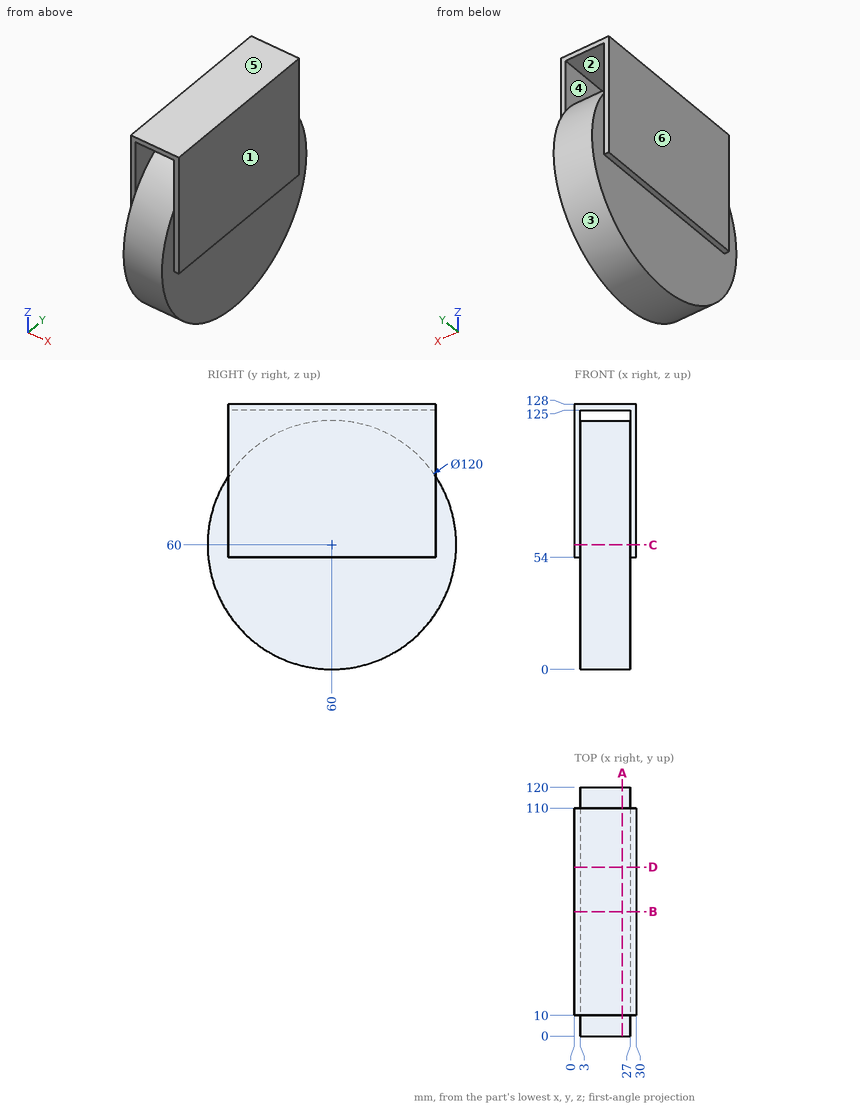
Design review of the part shown in the three views and the two pictorial views. Dimensions are in mm from the part's minimum x, y and z. A direction names the side the tool comes from. Give positions to 0.01 mm unless a question says otherwise; leave off trailing zeros. Write each loop counter-clockwise with the first axis right and the second up, starting at its lowest first coordinate (ties: lowest second). Pieces come first, ordered by that corner, then holes. Notation, with made-up numbers: (72.5, 22) - (81.5, 22) arc R19 ccw to (81.5, 30) - close; hole circle Ø10 at (74.25, 24.25). An arc over 180 degrees is marked (long way). Return JSON: item names as keys, results as strings. Group by question number.
(1) Insertion check: pin 1 (12 mm diameter, centred on x = 23.5, z = 107, fed in from -Y); pin 2 (8 mm diameter, centred on x = 24, y = 72.5, fed in from -Z); pin 3 (3.5 mm diameter, centred on x = 2, y = 54.5, fed in from -Z). Each pin has a flat end and moves straight along its axis. Give the tip position at first contact, or say it passes through.
(2) Mouldability with a two-part tool opening along X and no side actions: class the marked faces 4, 5 and 6 as +X half, -X half, draft (parallel to the pull), parting line (faces both ways), or undercut.
(3) We need section C-C, the plane z = 60. Give the boundary of the cut face in (x, y).
(4) We need section A-A, the plane x = 23.25. Give the boundary of the cut face in (y, z).
(5) Machinability: for the marked faces 1, 2 and 3, which of the approach directions +Z, -Z, +X, -X, +Y, -Y give a long, thin tool a straight path to every point of the face, cutting with its end or side? Answer none if there is none.
(6) We need section B-B, the plane y = 60. Give the boundary of the cut face in (x, z).
(7) To check wall thickness, follow probe 1 along X at (y, z) = (30.5, 115.5); probe 2 along Z at (x, y) = (11, 34.5); probe 3 along Z at (x, y) = (28.75, 12). State the ranges of each line that lie inside material, in increasing order.
(8) We need section D-D, the plane y = 81.5. Give the boundary of the cut face in (x, z).
Reported:
{
 "1": {"pin 1": "stops at y = 10", "pin 2": "stops at z = 0.61", "pin 3": "stops at z = 0.14"},
 "2": {"face 4": "undercut", "face 5": "draft", "face 6": "-X half"},
 "3": {"outline": "(0, 10) - (3, 10) - (3, 0) - (27, 0) - (27, 10) - (30, 10) - (30, 110) - (27, 110) - (27, 120) - (3, 120) - (3, 110) - (0, 110) - close"},
 "4": {"outline": "circle Ø120 at (60, 60); (10, 125) - (110, 125) - (110, 128) - (10, 128) - close"},
 "5": {"face 1": "+Z, -Z, +X, +Y, -Y", "face 2": "+Y, -Y", "face 3": "none"},
 "6": {"outline": "(0, 54) - (3, 54) - (3, 0) - (27, 0) - (27, 54) - (30, 54) - (30, 128) - (0, 128) - close; hole (3, 120) - (27, 120) - (27, 125) - (3, 125) - close"},
 "7": {"probe 1": "x = 0 to 3, 27 to 30", "probe 2": "z = 5.69 to 114.31, 125 to 128", "probe 3": "z = 54 to 128"},
 "8": {"outline": "(0, 54) - (3, 54) - (3, 3.98) - (27, 3.98) - (27, 54) - (30, 54) - (30, 128) - (0, 128) - close; hole (3, 116.02) - (27, 116.02) - (27, 125) - (3, 125) - close"}
}
